Source: CAD feature listing. Evaluate the final solid. Frame: model axes, mm. A direction names the side the tool comes from. Give positions to 0.01 mm unless a question says otherwise; leave off trailing zeros. Order: outer loops, then holes, each group sorted by start corner. A loop starts at its lowest first (then second) coordinate and runs counter-clockwise, first axis right, second up.
```python
from build123d import *

# Parameters (mm, degrees)
CYLINDER006_R           = 1.45
CYLINDER006_DEPTH       = 50
CYLINDER007_R           = 1.45
CYLINDER007_DEPTH       = 50
BODY007_PLACEMENT_ANGLE = 15
BOX_W                   = 226
BOX_H                   = 17
BOX_DEPTH               = 3
PAD005_DEPTH            = 180
BODY011_PITCH_ANGLE     = -90
BODY011_PLACEMENT_ANGLE = -90


with BuildPart() as cylinder004:
    # Cylinder006 → Cylinder006 (new body)
    with BuildSketch(Plane(origin=(23, 5, -5), x_dir=(1, 0, 0), z_dir=(0, 0, 1))):
        Circle(CYLINDER006_R)
    extrude(amount=CYLINDER006_DEPTH)


with BuildPart() as round_holes_clone:
    # Cylinder007 → Cylinder007 (new body)
    with BuildSketch(Plane(origin=(21, 12, -5), x_dir=(1, 0, 0), z_dir=(0, 0, 1))):
        Circle(CYLINDER007_R)
    extrude(amount=CYLINDER007_DEPTH)

    # Fusion: union Cylinder004
    add(cylinder004.part)


with BuildPart() as round_holes_clone_1:
    # Body007 placement: moved
    add(round_holes_clone.part.moved(Location((0, 5.95964, -31))).rotate(Axis((0, 5.95964, -31), (0, 0, -1)), BODY007_PLACEMENT_ANGLE))


with BuildPart() as fusion003:
    # Part__Mirroring001: instance of round holes clone
    add(round_holes_clone_1.part.mirror(Plane(origin=(132, 0, 0), x_dir=(0, -1, 0), z_dir=(1, 0, 0))))

    # Fusion003: union round holes clone
    add(round_holes_clone_1.part)


with BuildPart() as fusion003_1:
    # Fusion003 placement: moved
    add(fusion003.part.moved(Location((-18, 0, 0))))


with BuildPart() as body009:
    # Box → Box (new body)
    with BuildSketch(Plane.XY):
        with Locations((113, 8.5)):
            Rectangle(BOX_W, BOX_H)
    extrude(amount=BOX_DEPTH)

    # Cut003: cut Fusion003
    add(fusion003_1.part, mode=Mode.SUBTRACT)


with BuildPart() as fusion004:
    # Sketch005 → Pad005 (new body)
    with BuildSketch(Plane.XZ):
        with BuildLine():
            Line((-8.5, -3), (-8.5, 20))
            Line((-8.5, 20), (-5.5, 20))
            add(Edge.make_bspline(
                [(-5.5, 20), (-5.5, 1.17), (0, 0), (5.5, 1.17), (5.5, 6)],
                knots=[0, 0, 0, 0, 0.5, 1, 1, 1, 1], degree=3))
            Line((5.5, 6), (7.5, 6))
            Line((7.5, 6), (7.5, -3))
            Line((7.5, -3), (-8.5, -3))
        make_face()
    extrude(amount=PAD005_DEPTH)


with BuildPart() as fusion004_1:
    # Body011 pitch: moved
    add(fusion004.part.rotate(Axis((0, 0, 0), (0, 1, 0)), BODY011_PITCH_ANGLE))


with BuildPart() as fusion004_2:
    # Body011 placement: moved
    add(fusion004_1.part.moved(Location((203, 3, 8.5))).rotate(Axis((203, 3, 8.5), (0, 0, 1)), BODY011_PLACEMENT_ANGLE))

    # Fusion004: union Body009
    add(body009.part)


solid = fusion004_2.part
```
1) Pin query (flat end, axial travel): pin 1 (2.5 mm diameter, centred on x = 212.5, z = 2, fed in from +Y); pin 2 (6 mm diameter, centred on x = 201, y = 17, fed in from +Z); pin 3 (4 mm diameter, centred on x = 222.61, y = 12.12, fed in from +Z). Return the tip coordinate at first contact, or that it passes through.
Report:
pin 1: stops at y = 17
pin 2: stops at z = 3.29
pin 3: stops at z = 3
2) Section query A-A, the plane x = 211. Return the cut outline in (y, z).
Report:
outline: (0, 0) - (17, 0) - (17, 3) - (0, 3) - close
3) Material intervals for L1, parallel to Y at x = 34, z = 6.5; L2, parallel to X at y = 2.75, z = 5.5; L3, parallel to Z at x = 110, y = 19.25, sorted ascending.
Report:
L1: y = 0 to 3.96
L2: x = 23 to 203
L3: z = 0 to 3.04
4) Reachability of faces 1 (the flat face through (11, 9, 3)), 2 (the flat face through (214, 9, 3)), 3 (the flat face through (111, 12, 0)) from +Z, -Z, +X, -X, +Y, -Y: full face, straight path, thin tool, end or side. Return the list, or none.
Report:
face 1: +Z, -X, +Y, -Y
face 2: +Z, +X, +Y, -Y
face 3: -Z, +X, -X, +Y, -Y
